from build123d import *

# Parameters (mm, degrees)
SKETCH1_W           = 8
SKETCH1_H           = 13
BOSS_EXTRUDE1_DEPTH = 12
SKETCH2_W           = 13
SKETCH2_H           = 5
CUT_EXTRUDE1_DEPTH  = 7
SKETCH3_R           = 1
CUT_EXTRUDE2_DEPTH  = 19.138357147
CUT_EXTRUDE3_START  = -13
CUT_EXTRUDE3_DEPTH  = 32.138357147
SKETCH7_W           = 8
SKETCH7_H           = 3.5
BOSS_EXTRUDE4_DEPTH = 10


with BuildPart() as part:
    # Sketch1 → Boss-Extrude1 (new body)
    with BuildSketch(Plane(origin=(0, 0, 0), x_dir=(1, 0, 0), z_dir=(0, 1, 0))):
        Rectangle(SKETCH1_W, SKETCH1_H)
    extrude(amount=BOSS_EXTRUDE1_DEPTH)

    # Sketch2 → Cut-Extrude1 (cut)
    with BuildSketch(Plane(origin=(0, 12, 0), x_dir=(1, 0, 0), z_dir=(0, 1, 0))):
        Rectangle(SKETCH2_W, SKETCH2_H)
    extrude(amount=-CUT_EXTRUDE1_DEPTH, mode=Mode.SUBTRACT)

    # Sketch3 → Cut-Extrude2 (cut, through all)
    with BuildSketch(Plane(origin=(0, 0, -6.5), x_dir=(-1, 0, 0), z_dir=(0, 0, -1))):
        with Locations((0, 8)):
            Circle(SKETCH3_R)
    extrude(amount=-CUT_EXTRUDE2_DEPTH, mode=Mode.SUBTRACT)

    # Sketch4 → Cut-Extrude3 (cut)
    with BuildSketch(Plane(origin=(0, 0, -6.5), x_dir=(-1, 0, 0), z_dir=(0, 0, -1)).offset(CUT_EXTRUDE3_START)):
        with BuildLine():
            Line((-4, -27.298221281), (-4, 8))
            ThreePointArc((-4, 8), (-2.828427125, 10.828427125), (0, 12))
            Line((0, 12), (35.298221281, 12))
            Line((35.298221281, 12), (-14.621001982, 61.919223264))
            Line((-14.621001982, 61.919223264), (-53.919223264, 22.621001982))
            Line((-53.919223264, 22.621001982), (-4, -27.298221281))
        make_face()
    cut_extrude3 = extrude(amount=CUT_EXTRUDE3_DEPTH, mode=Mode.SUBTRACT)

    # Mirror1: Cut-Extrude3 across plane
    add(cut_extrude3.mirror(Plane(origin=(0, 0, 0), x_dir=(0, 0, 1), z_dir=(1, 0, 0))), mode=Mode.SUBTRACT)

    # Sketch7 → Boss-Extrude4 (add)
    with BuildSketch(Plane.XZ):
        with Locations((0, -4.75)):
            Rectangle(SKETCH7_W, SKETCH7_H)
    boss_extrude4 = extrude(amount=BOSS_EXTRUDE4_DEPTH)

    # Mirror2: Boss-Extrude4 across plane
    add(boss_extrude4.mirror(Plane.XY))


solid = part.part
Model file for the job. Use its own axes, mm. A direction names the side the tool comes from. Give positions to 0.01 mm unless a question says otherwise; leave off trailing zeros. Order: outer loops, then holes, each group sorted by start corner. A loop starts at its lowest first (then second) coordinate and runs counter-clockwise, first axis right, second up. Notation, with made-up numbers: (13.25, 14) -> (19.25, 14) arc R22 cw to (19.25, 42) -> close; hole circle Ø7 at (-24, 13.5). An arc over 180 degrees is marked (long way). Use CSV: the item, a comma, the result in double quotes.
1. 3-axis set-ups, long thin cutter, end or side, ignore diameter. For faces 1 (the flat face through (-1, 9, -2.5)), 2 (the cylindrical face through (0, 9, 4)), 3 (the flat face through (0, 0, 0)): which of +Z, -Z, +X, -X, +Y, -Y reach the whole face in a straight line?
Outcome:
face 1,"+X, -X, +Y"
face 2,"+Z, -Z"
face 3,"+X, -X, -Y"
2. Band-saw the part on B-B, the plane x = 0.5. Give the cut face in (y, z), then the cut area to 3 significant figures.
Outcome:
outline,"(-10, -6.5) -> (7.13, -6.5) -> (7.13, -2.5) -> (5, -2.5) -> (5, 2.5) -> (7.13, 2.5) -> (7.13, 6.5) -> (-10, 6.5) -> (-10, 3) -> (0, 3) -> (0, -3) -> (-10, -3) -> close; (8.87, -6.5) -> (11.97, -6.5) -> (11.97, -2.5) -> (8.87, -2.5) -> close; (8.87, 2.5) -> (11.97, 2.5) -> (11.97, 6.5) -> (8.87, 6.5) -> close"
area,"177 mm²"
3. Band-saw the part on D-D, the plane y = -6. Give the cut face in (x, z).
Outcome:
outline,"(-4, -6.5) -> (4, -6.5) -> (4, -3) -> (-4, -3) -> close; (-4, 3) -> (4, 3) -> (4, 6.5) -> (-4, 6.5) -> close"
4. Band-saw the part on C-C, the plane z = -4.75. Give the cut face in (x, y), then the cut area to 3 significant figures.
Outcome:
outline,"(-4, -10) -> (4, -10) -> (4, 8) arc R4 ccw to (-4, 8) -> close; hole circle Ø2 at (0, 8)"
area,"166 mm²"
5. Mould opens along Z. For faces 4 (the flat face through (0, 1, 6.5)), 5 (the flat face through (0, 5, 0)), 6 (the flat face through (-4, 1, 0)) say: +Z half, -Z half, draft (parallel to the pull), parting line (faces both ways), or undercut.
Outcome:
face 4,"+Z half"
face 5,"undercut"
face 6,"draft"
6. Drill centre lines: line 1 along Y through (x, z) = (0, 3.65); line 2 along Z through (x, y) = (-2.25, -2.5); line 3 along Z through (x, y) = (-3, 10). Where is each one in solid material? Low to high. Write a range as from..to.
Outcome:
line 1,"-10..7, 9..12"
line 2,"-6.5..-3, 3..6.5"
line 3,"-6.5..-2.5, 2.5..6.5"
7. Drop flat-ended pins along their axis: pin 1 (3 mm diameter, centred on x = -1, z = 0, fed in from -Y); pin 2 (4 mm diameter, centred on x = -0.5, z = 0, fed in from +Y). Give the stop position or say it passes through.
Outcome:
pin 1,"y = 0"
pin 2,"y = 5"
8. Band-saw the part on A-A, the plane y = 5.5. Give the cut face in (x, z), then the cut area to 3 significant figures.
Outcome:
outline,"(-4, -6.5) -> (4, -6.5) -> (4, -2.5) -> (-4, -2.5) -> close; (-4, 2.5) -> (4, 2.5) -> (4, 6.5) -> (-4, 6.5) -> close"
area,"64.0 mm²"
